Source: CAD feature listing. Evaluate the final solid. Frame: model axes, mm. Face numbers are marked on the shaded views. A direction names the side the tool comes from. Give positions to 0.01 mm unless a question says otherwise; leave off trailing zeros. Write each loop counter-clockwise with the first axis right and the second up, starting at its lowest first coordinate (ties: lowest second). Pieces come first, ordered by that corner, then holes. Notation, with made-up numbers: M 25.5,-36.75 L 50.5,-36.75 A21 cw 50.5,-18.75 Z; hole C 18,34.5 d10. An arc over 180 degrees is marked long. Use CSV: the item, a comma, the result in double quotes. Start each with the question number.
from build123d import *

# Parameters (mm, degrees)
BOSS_EXTRUDE1_DEPTH = 104.775
BOSS_EXTRUDE2_DEPTH = 92.5957
BOSS_EXTRUDE3_START = -5.8293
BOSS_EXTRUDE3_DEPTH = 5.8293
BOSS_EXTRUDE4_DEPTH = 6.35
SKETCH5_W           = 7.787485422
SKETCH5_H           = 19.833751934
SKETCH5_W_2         = 22.754058967
SKETCH5_H_2         = 3.407024872
CUT_EXTRUDE1_DEPTH  = 227.312030137
FILLET1_R           = 6.35
SKETCH6_R           = 6.35
CUT_EXTRUDE2_DEPTH  = 6.35


with BuildPart() as part:
    # Sketch1 → Boss-Extrude1 (new, symmetric)
    with BuildSketch(Plane.XY):
        with BuildLine():
            Line((-58.2422, 56.2102), (-58.2422, 62.5602))
            ThreePointArc((-58.2422, 62.5602), (-45.640852469, 57.743322347), (-39.3748699, 45.7962))
            ThreePointArc((-39.3748699, 45.7962), (-25.556268964, 20.239931036), (0, 6.4213301))
            ThreePointArc((0, 6.4213301), (12.247457496, 0.293755183), (17.272, -12.446))
            Line((17.272, -12.446), (10.922, -12.446))
            ThreePointArc((10.922, -12.446), (7.760938146, -4.204686933), (0, 0))
            ThreePointArc((0, 0), (-30.011530905, 15.784669095), (-45.7962, 45.7962))
            ThreePointArc((-45.7962, 45.7962), (-50.144819563, 53.243313205), (-58.2422, 56.2102))
        make_face()
    extrude(amount=BOSS_EXTRUDE1_DEPTH, both=True)


with BuildPart() as boss_extrude2_tool:
    # Sketch2 → Boss-Extrude2 (new, symmetric)
    with BuildSketch(Plane.XY):
        with BuildLine():
            Line((-58.2422, 56.2102), (-58.2422, 45.796198296))
            Line((-58.2422, 45.796198296), (-45.796199685, 45.796198296))
            ThreePointArc((-45.796199685, 45.796198296), (-50.144818899, 53.243312648), (-58.2422, 56.2102))
        make_face()
        with BuildLine():
            Line((0, 0), (0, -12.446))
            Line((0, -12.446), (10.922, -12.446))
            ThreePointArc((10.922, -12.446), (7.760938146, -4.204686933), (0, 0))
        make_face()
    extrude(amount=BOSS_EXTRUDE2_DEPTH, both=True)


with BuildPart() as part_1:
    add(part.part)


with BuildPart() as part_2:
    # Boss-Extrude2: joined with boss_extrude2_tool
    add(part_1.part.fuse(boss_extrude2_tool.part, tol=0.00001))

    # Sketch3 → Boss-Extrude3 (add)
    with BuildSketch(Plane(origin=(0, 0, -104.775), x_dir=(-1, 0, 0), z_dir=(0, 0, -1)).offset(BOSS_EXTRUDE3_START)):
        with BuildLine():
            Line((58.2422, 56.2102), (58.2422, 45.796198296))
            Line((58.2422, 45.796198296), (45.7962, 45.7962))
            ThreePointArc((45.7962, 45.7962), (50.144819563, 53.243313205), (58.2422, 56.2102))
        make_face()
        with BuildLine():
            Line((0, 0), (0, -12.446))
            Line((0, -12.446), (-10.922, -12.446))
            ThreePointArc((-10.922, -12.446), (-7.760938146, -4.204686933), (0, 0))
        make_face()
    extrude(amount=BOSS_EXTRUDE3_DEPTH)

    # Sketch4 → Boss-Extrude4 (add)
    with BuildSketch(Plane.XY.offset(104.775)):
        with BuildLine():
            Line((-58.2422, 56.2102), (-58.2422, 45.796198296))
            Line((-58.2422, 45.796198296), (-45.7962, 45.7962))
            ThreePointArc((-45.7962, 45.7962), (-50.144819563, 53.243313205), (-58.2422, 56.2102))
        make_face()
        with BuildLine():
            Line((0, 0), (0, -12.446))
            Line((0, -12.446), (10.922, -12.446))
            ThreePointArc((10.922, -12.446), (7.760938146, -4.204686933), (0, 0))
        make_face()
    extrude(amount=-BOSS_EXTRUDE4_DEPTH)

    # Sketch5 → Cut-Extrude1 (cut, through all)
    with BuildSketch(Plane.XY.offset(104.775)):
        with Locations((-61.627942711, 54.680509116)):
            Rectangle(SKETCH5_W, SKETCH5_H)
        with Locations((8.225058429, -13.641512436)):
            Rectangle(SKETCH5_W_2, SKETCH5_H_2)
    extrude(amount=-CUT_EXTRUDE1_DEPTH, mode=Mode.SUBTRACT)

    # Fillet1
    # the kernel refuses this fillet: 6.35 mm, written as the material it takes off along each edge
    with BuildSketch(Plane(origin=(17.260151367, -11.938, -130.624178653), x_dir=(-0.30497213299383213, 0.9523612749882223, 0), z_dir=(0, 0, 1))) as fillet1_piece_1:
        with BuildLine():
            CenterArc((8.625598356, 6.114282737), FILLET1_R, 162.243512631, 123.416753829)
            Line((2.57810426, 8.050855782), (0, 0))
            ThreePointArc((0, 0), (5.169835731, -0.710949564), (10.339671461, 0))
        make_face()
    extrude(amount=261.248357306, mode=Mode.SUBTRACT)
    with BuildSketch(Plane(origin=(-57.7342, 62.551510856, -130.462315531), x_dir=(0.9544368882494849, -0.29841284548196007, 0), z_dir=(0, 0, 1))) as fillet1_piece_2:
        with BuildLine():
            CenterArc((8.565200947, -6.11549994), FILLET1_R, 74.380472255, 122.981827606)
            Line((2.504526706, -8.010421509), (0, 0))
            ThreePointArc((0, 0), (5.137463106, 0.704636839), (10.274926212, 0))
        make_face()
    extrude(amount=260.924631062, mode=Mode.SUBTRACT)

    # Sketch6 → Cut-Extrude2 (cut, symmetric)
    with BuildSketch(Plane(origin=(-5.969, -5.969000176, 0), x_dir=(-0.7071067916239179, 0.7071067707491772, 0), z_dir=(-0.7071067707491772, -0.7071067916239179, 0))):
        with Locations(Location((32.382802858, 75.980128158, 0), (0, 0, 180))):
            Circle(SKETCH6_R)
    extrude(amount=CUT_EXTRUDE2_DEPTH, both=True, mode=Mode.SUBTRACT)


solid = part_2.part
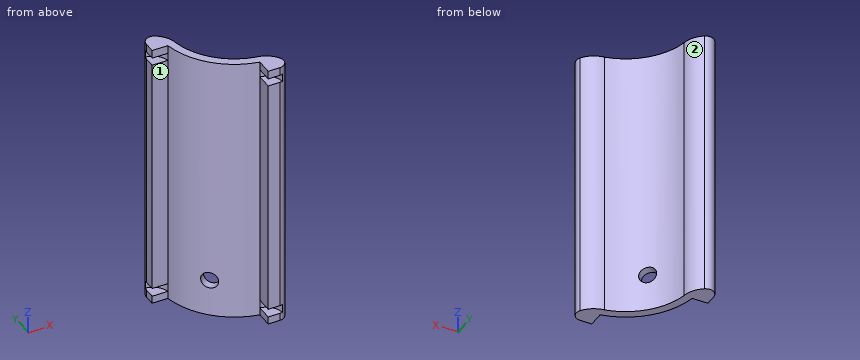
1. Section D-D on y = 32. Return loops of the section in (x, z) (3 decimals).
2. Line query: probe 1 along Z at (x, y) = (8, -5) (3 decimals); probe 2 along Y at (x, z) = (-13, 19); probe 3 along X at (y, z) = (44, -87.5). Output: solid intervals per line, ascending.
3. Section B-B on z = -78. Return loops of the section in (x, y), then the cut area to 3 significant figures.
4. First-contact query: pin 1 (7 mm diameter, centred on y = -4.5, z = 102, fed in from -X); pin 2 (9.5 mm diameter, centred on x = -54, z = -9, fed in from -Y); pin 3 (4 mm diameter, centred on y = 14.5, z = -1, fed in from -X). Flat tips, straight axial feed; report the tip coordinate or a pass-through.
5. Section C-C on x = -2.5. Return loops of the section in (y, z) (3 decimals), then the cut area to 3 significant figures.
6. Section A-A on z = 40. Return loops of the section in (x, y).
7. Access query for the marked faces 1 and 2. Directions: +Z, -Z, +X, -X, +Y, -Y. A direction counts if a zero-diameter tool reaches every point of the face in a straight line with its end or side. Return the directions, or none.
Resolved:
1,outline,"M -41.376,-104.775 L -34.324,-104.775 L -34.324,104.775 L -41.376,104.775 Z"
2,probe 1,"z = -104.775 to -98.946, -92.596 to 92.596, 98.425 to 104.775"
2,probe 2,"y = 4.06 to 11.05"
2,probe 3,"x = -45.43 to -38.97"
3,outline,"M -57.73,45.8 L -45.8,45.8 A57.15 ccw -34.04,20.27 L -29.56,24.75 A50.85 cw -39.37,45.8 A19.08 ccw -47.93,59.49 A6.35 ccw -57.73,54.16 Z; M -25.53,11.75 A57.15 ccw 0,0 L 0,-11.94 L 8.81,-11.94 A6.35 ccw 14.11,-2.09 A19.15 ccw 0,6.42 A50.85 cw -21.05,16.24 Z"
3,area,"759 mm2"
4,pin 1,"stops at x = 0"
4,pin 2,"stops at y = 45.8"
4,pin 3,"stops at x = -30.71"
5,outline,"M 0.521,-104.775 L 7.01,-104.775 L 7.01,104.775 L 0.521,104.775 Z"
5,area,"1,360 mm2"
6,outline,"M -57.73,45.8 L -45.8,45.8 A57.15 ccw 0,0 L 0,-11.94 L 8.81,-11.94 A6.35 ccw 14.11,-2.09 A19.15 ccw 0,6.42 A50.85 cw -39.37,45.8 A19.08 ccw -47.93,59.49 A6.35 ccw -57.73,54.16 Z"
7,face 1,"+Z, -Z, -X, -Y"
7,face 2,"+Z, -Z, +X, +Y"
